Could you check a few things on this model? Use its own coordinates, in mm. A direction names the side the tool comes from. Round coordinates to 2 decimals unless told otherwise and drop trailing zeros. Loops run counter-clockwise (first coordinate to the right, second up) from the corner with the lowest first, then second, coordinate; pieces in that order, holes last. Notation, with made-up numbers: (82, 78) - (137, 78) arc R14 cw to (137, 89) - close; hole circle Ø10 at (-8, 20.25). An arc over 180 degrees is marked (long way). Use one line per item in the form item = value.
```python
from build123d import *

# Parameters (mm, degrees)
SKETCH1_R               = 3.96875
BOSS_EXTRUDE1_DEPTH     = 9.525
BOSS_EXTRUDE4_START     = 9.525
BOSS_EXTRUDE4_OUTLINE_R = 3.96875
BOSS_EXTRUDE4_DEPTH     = 15.875
BOSS_EXTRUDE5_START     = 25.4
BOSS_EXTRUDE5_DEPTH     = 38.1
SKETCH4_R               = 9.525
CUT_EXTRUDE1_DEPTH      = 177.01216089
SKETCH2_R               = 9.525
SKETCH2_W               = 12.7
SKETCH2_H               = 28.575
CUT_EXTRUDE2_DEPTH      = 182.288051609
CUT_EXTRUDE3_DEPTH      = 3.175
CUT_EXTRUDE4_START      = -12.7
CUT_EXTRUDE4_DEPTH      = 7.9375


# Read off the part's stored shape, not the designer's step: Boss-Extrude4, Boss-Extrude5
with BuildPart() as part:
    # Sketch1 → Boss-Extrude1 (new body)
    with BuildSketch(Plane.XY):
        with BuildLine():
            Line((0, 0), (92.075, 0))
            ThreePointArc((92.075, 0), (96.565128061, -1.859871939), (98.425, -6.35))
            Line((98.425, -6.35), (98.425, -12.7))
            ThreePointArc((98.425, -12.7), (109.5375, -23.8125), (120.65, -12.7))
            Line((120.65, -12.7), (120.65, -6.35))
            ThreePointArc((120.65, -6.35), (122.509871939, -1.859871939), (127, 0))
            Line((127, 0), (139.7, 0))
            Line((139.7, 0), (139.7, -7.9375))
            Line((139.7, -7.9375), (165.1, -7.9375))
            Line((165.1, -7.9375), (165.1, 12.7))
            Line((165.1, 12.7), (139.7, 12.7))
            Line((139.7, 12.7), (139.7, 9.525))
            Line((139.7, 9.525), (80.01, 9.525))
            ThreePointArc((80.01, 9.525), (77.315923164, 10.640923164), (76.2, 13.335))
            Line((76.2, 13.335), (76.2, 28.575))
            Line((76.2, 28.575), (61.9125, 28.575))
            Line((61.9125, 28.575), (61.9125, 44.45))
            Line((61.9125, 44.45), (53.975, 44.45))
            Line((53.975, 44.45), (53.975, 13.335))
            ThreePointArc((53.975, 13.335), (52.859076836, 10.640923164), (50.165, 9.525))
            Line((50.165, 9.525), (9.525, 9.525))
            Line((9.525, 9.525), (9.525, 52.3875))
            Line((9.525, 52.3875), (0, 52.3875))
            Line((0, 52.3875), (0, 0))
        make_face()
        with Locations(Location((109.5375, -12.7, 0), (0, 0, 180))):
            Circle(SKETCH1_R, mode=Mode.SUBTRACT)
        with Locations(Location((65.0875, 19.05, 0), (0, 0, 180))):
            Circle(SKETCH1_R, mode=Mode.SUBTRACT)
    extrude(amount=BOSS_EXTRUDE1_DEPTH)

    # Boss-Extrude4 outline → Boss-Extrude4 (add)
    with BuildSketch(Plane.XY.offset(BOSS_EXTRUDE4_START)):
        with BuildLine():
            Line((9.525, 52.3875), (0, 52.3875))
            Line((0, 52.3875), (0, 0))
            Line((0, 0), (139.7, 0))
            Line((139.7, 0), (139.7, -7.9375))
            Line((139.7, -7.9375), (165.1, -7.9375))
            Line((165.1, -7.9375), (165.1, 12.7))
            Line((165.1, 12.7), (139.7, 12.7))
            Line((139.7, 12.7), (139.7, 9.525))
            Line((139.7, 9.525), (80.01, 9.525))
            ThreePointArc((80.01, 9.525), (77.315923164, 10.640923164), (76.2, 13.335))
            Line((76.2, 13.335), (76.2, 28.575))
            Line((76.2, 28.575), (61.9125, 28.575))
            Line((61.9125, 28.575), (61.9125, 44.45))
            Line((61.9125, 44.45), (53.975, 44.45))
            Line((53.975, 44.45), (53.975, 13.335))
            ThreePointArc((53.975, 13.335), (52.859076836, 10.640923164), (50.165, 9.525))
            Line((50.165, 9.525), (9.525, 9.525))
            Line((9.525, 9.525), (9.525, 52.3875))
        make_face()
        with Locations((65.0875, 19.05)):
            Circle(BOSS_EXTRUDE4_OUTLINE_R, mode=Mode.SUBTRACT)
    extrude(amount=BOSS_EXTRUDE4_DEPTH)

    # Boss-Extrude5 outline → Boss-Extrude5 (add)
    with BuildSketch(Plane.XY.offset(BOSS_EXTRUDE5_START)):
        Polygon((9.525, 52.3875), (0, 52.3875), (0, 0), (139.7, 0), (139.7, -7.9375), (165.1, -7.9375), (165.1, 12.7), (139.7, 12.7), (139.7, 9.525), (9.525, 9.525), align=None)
    extrude(amount=BOSS_EXTRUDE5_DEPTH)

    # Sketch4 → Cut-Extrude1 (cut, through all)
    with BuildSketch(Plane(origin=(9.525, 0, 0), x_dir=(0, 0, -1), z_dir=(1, 0, 0))):
        with BuildLine():
            Line((-63.5, 52.3875), (-63.5, 33.3375))
            ThreePointArc((-63.5, 33.3375), (-57.920384182, 46.807884182), (-44.45, 52.3875))
            Line((-44.45, 52.3875), (-63.5, 52.3875))
        make_face()
        with Locations(Location((-44.45, 33.3375, 0), (0, 0, 90))):
            Circle(SKETCH4_R)
    extrude(amount=-CUT_EXTRUDE1_DEPTH, mode=Mode.SUBTRACT)

    # Sketch2 → Cut-Extrude2 (cut, through all)
    with BuildSketch(Plane(origin=(0, 12.7, 0), x_dir=(1, 0, 0), z_dir=(0, 1, 0))):
        with Locations(Location((41.275, -44.45, 0), (0, 0, 180))):
            Circle(SKETCH2_R)
        with BuildLine():
            ThreePointArc((123.825, -63.5), (115.455576272, -43.294423728), (95.25, -34.925))
            ThreePointArc((95.25, -34.925), (75.044423728, -43.294423728), (66.675, -63.5))
            Line((66.675, -63.5), (123.825, -63.5))
        make_face()
        with BuildLine():
            ThreePointArc((66.675, -63.5), (95.25, -92.075), (123.825, -63.5))
            Line((123.825, -63.5), (66.675, -63.5))
        make_face()
        with BuildLine():
            Line((139.7, -63.5), (139.7, -34.925))
            Line((139.7, -34.925), (95.25, -34.925))
            ThreePointArc((95.25, -34.925), (115.455576272, -43.294423728), (123.825, -63.5))
            Line((123.825, -63.5), (139.7, -63.5))
        make_face()
        with BuildLine():
            Line((165.1, -63.5), (165.1, -22.225))
            ThreePointArc((165.1, -22.225), (161.380256121, -31.205256121), (152.4, -34.925))
            Line((152.4, -34.925), (152.4, -63.5))
            Line((152.4, -63.5), (165.1, -63.5))
        make_face()
        with Locations((146.05, -49.2125)):
            Rectangle(SKETCH2_W, SKETCH2_H)
        with BuildLine():
            Line((165.1, 0), (152.4, 0))
            Line((152.4, 0), (152.4, -9.525))
            ThreePointArc((152.4, -9.525), (161.380256121, -13.244743879), (165.1, -22.225))
            Line((165.1, -22.225), (165.1, 0))
        make_face()
        Polygon((152.4, -9.525), (152.4, 0), (139.7, 0), (139.7, -7.853947368), align=None)
        Polygon((139.7, -7.853947368), (139.7, 0), (80.01, 0), align=None)
        with BuildLine():
            ThreePointArc((158.75, -22.225), (156.890128061, -17.734871939), (152.4, -15.875))
            Line((152.4, -15.875), (152.4, -28.575))
            ThreePointArc((152.4, -28.575), (156.890128061, -26.715128061), (158.75, -22.225))
        make_face()
        with BuildLine():
            Line((152.4, -28.575), (152.4, -15.875))
            ThreePointArc((152.4, -15.875), (146.05, -22.225), (152.4, -28.575))
        make_face()
    extrude(amount=-CUT_EXTRUDE2_DEPTH, mode=Mode.SUBTRACT)

    # Sketch2<3> → Cut-Extrude3 (cut)
    with BuildSketch(Plane(origin=(0, 12.7, 0), x_dir=(1, 0, 0), z_dir=(0, 1, 0))):
        with BuildLine():
            ThreePointArc((152.4, -34.925), (143.419743879, -31.205256121), (139.7, -22.225))
            Line((139.7, -22.225), (139.7, -34.925))
            Line((139.7, -34.925), (152.4, -34.925))
        make_face()
        with BuildLine():
            ThreePointArc((139.7, -22.225), (143.419743879, -13.244743879), (152.4, -9.525))
            Line((152.4, -9.525), (139.7, -7.853947368))
            Line((139.7, -7.853947368), (139.7, -22.225))
        make_face()
    extrude(amount=-CUT_EXTRUDE3_DEPTH, mode=Mode.SUBTRACT)

    # Sketch2<5> → Cut-Extrude4 (cut)
    with BuildSketch(Plane(origin=(0, 12.7, 0), x_dir=(1, 0, 0), z_dir=(0, 1, 0)).offset(CUT_EXTRUDE4_START)):
        with BuildLine():
            ThreePointArc((139.7, -22.225), (143.419743879, -13.244743879), (152.4, -9.525))
            Line((152.4, -9.525), (139.7, -7.853947368))
            Line((139.7, -7.853947368), (139.7, -22.225))
        make_face()
        with BuildLine():
            ThreePointArc((152.4, -34.925), (143.419743879, -31.205256121), (139.7, -22.225))
            Line((139.7, -22.225), (139.7, -34.925))
            Line((139.7, -34.925), (152.4, -34.925))
        make_face()
    extrude(amount=-CUT_EXTRUDE4_DEPTH, mode=Mode.SUBTRACT)


solid = part.part
```
1. If we section it at B-B, the plane y = 5: Write out the boundary of the cut face in (x, z) (3 decimals), plus the area to 3 significant figures.
Solution:
outline = (0, 0) - (80.01, 0) - (152.4, 9.525) arc R12.7 ccw to (152.4, 34.925) - (95.25, 34.925) arc R28.575 cw to (66.675, 63.5) - (0, 63.5) - close; hole circle Ø19.05 at (41.275, 44.45); hole circle Ø12.7 at (152.4, 22.225)
area = 6,900 mm^2
2. If we section it at C-C, the plane z = 50: Write out the boundary of the cut face in (x, y) (1 decimal).
Solution:
outline = (0, 0) - (33.5, 0) - (33.5, 9.5) - (9.5, 9.5) - (9.5, 25.6) - (0, 25.6) - close; (0, 41.1) - (9.5, 41.1) - (9.5, 51.6) - (0, 51.6) - close; (49, 0) - (70.1, 0) - (70.1, 9.5) - (49, 9.5) - close
3. We'd pull the mould along Z, two halves only. Please class faces 1 (the face through (124, 5, 34.925)), 2 (the face through (61.912, 36, 13)), 3 (the face through (4.83, 38.46, 52.48)): +Z half, -Z half, draft (parallel to the pull), parting line (faces both ways), or undercut.
Solution:
face_1 = +Z half
face_2 = draft
face_3 = undercut
4. For P1, Ø6, axis at x = 84.5, z = 40.5, coming from the -Y side; P2, Ø12, axis at x = 82, z = 34.5, coming from the +Y side (3 decimals); P3, Ø5, axis at x = 138, y = 6, coming from the +Z side (3 decimals); P4, Ø2, axis at y = 44, z = 54.5, coming from the +X side (3 decimals), each with a flat end and sliding along its axis, tell me the tip position at first contact or that it passes through.
Solution:
P1 = through
P2 = 9.525
P3 = 34.925
P4 = 9.525
5. Please list where these lines run through material, in increasing order: line 1 along X through (y, z) = (19.05, 21.5) (3 decimals); line 2 along Y through (x, z) = (7, 44); line 3 along Y through (x, z) = (8, 15).
Solution:
line_1 = 0 to 9.525, 53.975 to 61.119, 69.056 to 76.2
line_2 = 0 to 23.82, 42.85 to 52.39
line_3 = 0 to 52.39
6. If we section it at A-A, the plane y = 19.05: Write out the boundary of the cut face in (x, z) (3 decimals).
Solution:
outline = (0, 0) - (9.525, 0) - (9.525, 63.5) - (0, 63.5) - close; (53.975, 0) - (61.119, 0) - (61.119, 25.4) - (53.975, 25.4) - close; (69.056, 0) - (76.2, 0) - (76.2, 25.4) - (69.056, 25.4) - close
7. On a 3-axis mill with a long thin cutter (end or side, diameter ignored), from which of +Z, -Z, +X, -X, +Y, -Y can I reach the whole of each face in a straight line? I mean faces 4 (the face through (120.65, -10, 7)), 5 (the face through (77, 11, 13)), 6 (the face through (69, 28.575, 13)), 7 (the face through (98.425, -9, 6)). Say none if no direction works.
Solution:
face_4 = +Z, -Z, +X, -Y
face_5 = +Z, -Z, +Y
face_6 = +Z, -Z, +X, +Y
face_7 = +Z, -Z, -X, -Y
